Can you work these out from the model? Positions are in its coordinate system, mm. Face numbers are marked on the shaded views. A direction names the side the tool comes from. Coordinates: 2 decimals unless noted, no trailing zeros. Order: outer loops, then holes, each group sorted by start corner. A loop starts at its lowest first (then second) coordinate and runs counter-clockwise, first axis right, second up. Notation, with made-up numbers: (63, 46.25) -> (118, 46.25) arc R7 ccw to (118, 59.25) -> close; hole circle Ø4 at (-32.75, -17). An arc over 180 degrees is marked (long way). Answer as a JSON object with one key per item and string values. Group by question number.
(1) For pin 1 (14 mm diameter, centred on x = -19.5, z = 24, fed in from +Y); pin 2 (9.5 mm diameter, centred on x = 4.5, y = 7.5, fed in from +Z); pin 3 (12 mm diameter, centred on x = 1, y = -11.5, fed in from +Z); pin 4 (6.5 mm diameter, centred on x = -7.5, z = 7.5, fed in from -Y), each with a flat end and sliding along its axis, tell me the tip position at first contact or that it passes through.
(2) I want a section at D-D, the plane x = -19. List the corners of the cut face in (y, z) for me.
(3) If we mould it in two halves opening along X, with no side actions, what happens to the marked faces 1, 2, 3 and 4? For each: pulls with the +X half, pulls with the -X half, needs draft (parallel to the pull), parting line crosses it, or undercut.
(4) I want a section at B-B, the plane z = 22. List the corners of the cut face in (x, y) for me.
(5) I want a section at C-C, the plane z = 12. List the corners of the cut face in (x, y) for me.
(6) I want a section at A-A, the plane y = -10.5. List the corners of the cut face in (x, z) for me.
(7) I need wall thicknesses on line 1 (X direction, y = -12.5, z = 14); line 2 (Z direction, x = -13, y = 8.5); line 3 (Y direction, x = 16.5, z = 30.5). Which ranges of each line are inside material? Lowest first, please.
(8) Which directions (+Z, -Z, +X, -X, +Y, -Y) give clear straight access to the entire face, cutting with the end or side of a thin tool? Please do the marked faces 5, 6 and 7.
Autodesk Inventor part; units mm, degrees
ref_plane "YZ Plane" through (0, 0, 0) normal (1, 0, 0) x (0, 1, 0)
ref_plane "XZ Plane" through (0, 0, 0) normal (0, 1, 0) x (-1, 0, 0)
ref_plane "XY Plane" through (0, 0, 0) normal (0, 0, 1) x (1, 0, 0)
sketch "Sketch1" plane through (0, 0, 0) normal (0, 0, 1) x (1, 0, 0)
  line L0 (-27.1073, 14.808) -> (23.6927, 14.808)
  line L1 (23.6927, 14.808) -> (23.6927, -16.942)
  line L2 (23.6927, -16.942) -> (-27.1073, -16.942)
  line L3 (-27.1073, -16.942) -> (-27.1073, 14.808)
  point P0 (0, 0)
  dimension "d0" = 50.8
  dimension "d1" = 31.75
extrude "Extrusion1" add sketch "Sketch1" along normal blind 31.75
sketch "Sketch2" plane through (0, 0, 31.75) normal (0, 0, 1) x (1, 0, 0)
  line L0 (-27.1073, -16.942) -> (23.6927, -16.942)
  line L1 (-14.4073, -16.942) -> (10.9927, -16.942)
  line L2 (10.9927, -16.942) -> (10.9927, 2.108)
  line L3 (10.9927, 2.108) -> (-14.4073, 2.108)
  line L4 (-14.4073, 2.108) -> (-14.4073, -16.942)
  line L5 (-27.1073, 14.808) -> (-27.1073, -16.942)
  line L6 (23.6927, -16.942) -> (23.6927, 14.808)
  point P0 (0, 0)
  dimension "d4" = 12.7
  dimension "d5" = 12.7
  dimension "d6" = 19.05
extrude "Extrusion2" cut sketch "Sketch2" against normal blind 31.75
sketch "Sketch3" plane through (23.6927, -16.942, 0) normal (1, 0, 0) x (0, 0, -1)
  line L0 (-31.75, 0) -> (-31.75, 31.75)
  line L1 (-31.75, 31.75) -> (-12.7, 31.75)
  line L2 (-12.7, 31.75) -> (-12.7, 12.7)
  line L3 (-12.7, 12.7) -> (-31.75, 12.7)
  line L4 (-31.75, 12.7) -> (-31.75, 31.75)
  point P0 (0, 16.942)
  dimension "d9" = 19.05
  dimension "d10" = 19.05
extrude "Extrusion3" cut sketch "Sketch3" against normal blind 50.8
properties part number "Figure 7_27_5"
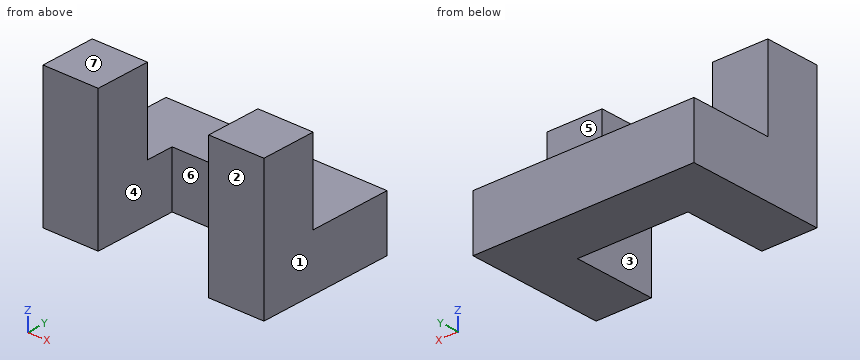
Computed values:
{
 "1": {"pin 1": "stops at y = -4.24", "pin 2": "stops at z = 12.7", "pin 3": "passes through", "pin 4": "stops at y = 2.11"},
 "2": {"outline": "(-16.94, 0) -> (14.81, 0) -> (14.81, 12.7) -> (-4.24, 12.7) -> (-4.24, 31.75) -> (-16.94, 31.75) -> close"},
 "3": {"face 1": "pulls with the +X half", "face 2": "needs draft", "face 3": "undercut", "face 4": "undercut"},
 "4": {"outline": "(-27.11, -16.94) -> (-14.41, -16.94) -> (-14.41, -4.24) -> (-27.11, -4.24) -> close; (10.99, -16.94) -> (23.69, -16.94) -> (23.69, -4.24) -> (10.99, -4.24) -> close"},
 "5": {"outline": "(-27.11, -16.94) -> (-14.41, -16.94) -> (-14.41, 2.11) -> (10.99, 2.11) -> (10.99, -16.94) -> (23.69, -16.94) -> (23.69, 14.81) -> (-27.11, 14.81) -> close"},
 "6": {"outline": "(-27.11, 0) -> (-14.41, 0) -> (-14.41, 31.75) -> (-27.11, 31.75) -> close; (10.99, 0) -> (23.69, 0) -> (23.69, 31.75) -> (10.99, 31.75) -> close"},
 "7": {"line 1": "x = -27.11 to -14.41, 10.99 to 23.69", "line 2": "z = 0 to 12.7", "line 3": "y = -16.94 to -4.24"},
 "8": {"face 5": "+Z, +X, -X, +Y", "face 6": "+Z, -Z, -Y", "face 7": "+Z, +X, -X, +Y, -Y"}
}
